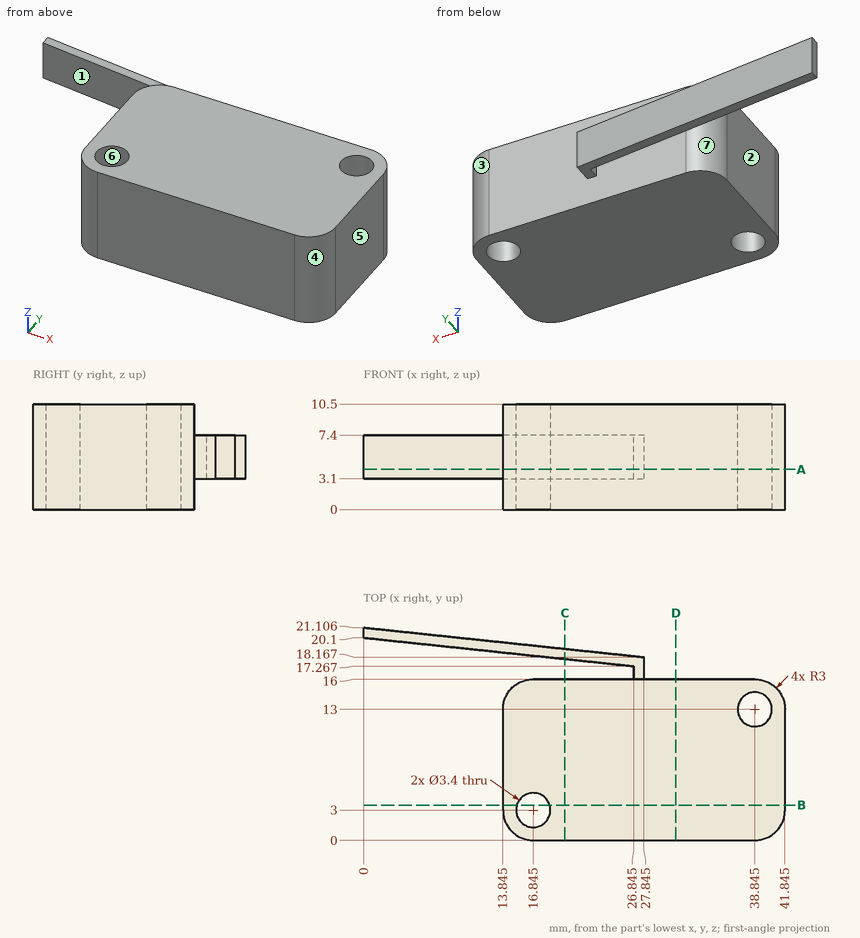
The figure shows three views and two pictorial views of one solid part (mm, origin at its lowest corner). Answer the questions. A direction names the side the tool comes from. Give positions to 0.01 mm unless a question says otherwise; leave off trailing zeros. Write each loop counter-clockwise with the first axis right and the second up, starting at its lowest first coordinate (ties: lowest second). Pieces come first, ordered by that corner, then holes. Notation, with made-up numbers: (-32, -24.75) -> (6, -24.75) arc R28 ccw to (6, -2.75) -> close; hole circle Ø9 at (-8, 48.25). An arc over 180 degrees is marked (long way). Answer as a JSON object with one key per item and string values.
1) Straight lines are drawn through the part: probe 1 along Y at (x, z) = (37, 4.5); probe 2 along Y at (x, z) = (26.5, 7); probe 3 along X at (y, z) = (13.75, 7.75). For each, find the intervals that lie inside material, in ascending order. Write a range as from..to.
Findings below:
{"probe 1": "y = 0..16", "probe 2": "y = 0..16, 17.3..18.31", "probe 3": "x = 13.94..37.32, 40.37..41.75"}
2) Section A-A on z = 4 is taken. Write down the section's boundary in (x, y) (1 decimal).
Findings below:
{"outline": "(0, 20.1) -> (26.8, 17.3) -> (26.8, 16) -> (16.8, 16) arc R3 ccw to (13.8, 13) -> (13.8, 3) arc R3 ccw to (16.8, 0) -> (38.8, 0) arc R3 ccw to (41.8, 3) -> (41.8, 13) arc R3 ccw to (38.8, 16) -> (27.8, 16) -> (27.8, 18.2) -> (0, 21.1) -> close; hole circle Ø3.4 at (16.8, 3); hole circle Ø3.4 at (38.8, 13)"}
3) Section D-D on x = 31 is taken. Write down the section's boundary in (y, z).
Findings below:
{"outline": "(0, 0) -> (16, 0) -> (16, 10.5) -> (0, 10.5) -> close"}
4) Section C-C on x = 20 is taken. Write down the section's boundary in (y, z) (1 decimal), then the cut area to 3 significant figures.
Findings below:
{"outline": "(0, 0) -> (16, 0) -> (16, 10.5) -> (0, 10.5) -> close; (18, 3.1) -> (19, 3.1) -> (19, 7.4) -> (18, 7.4) -> close", "area": "172 mm^2"}
5) Section B-B on y = 3.5 is taken. Write down the section's boundary in (x, z) (1 decimal).
Findings below:
{"outline": "(13.8, 0) -> (15.2, 0) -> (15.2, 10.5) -> (13.8, 10.5) -> close; (18.5, 0) -> (41.8, 0) -> (41.8, 10.5) -> (18.5, 10.5) -> close"}
6) A tool of negligible diameter and unlimited length cuts with its end or side. For the marked faces 1, 2 and 3, from which of +Z, -Z, +X, -X, +Y, -Y can it reach the whole face along a straight path? Write none if from no direction.
Findings below:
{"face 1": "+Z, -Z, -X", "face 2": "+Z, -Z, -X, -Y", "face 3": "+Z, -Z, +X, +Y"}
7) For a pull along Y with two mould halves and no side action, classify the marked faces 4, 5, 6 and 7 as pulls with the +Y half, pulls with the -Y half, needs draft (parallel to the pull), parting line crosses it, or undercut.
Findings below:
{"face 4": "pulls with the -Y half", "face 5": "needs draft", "face 6": "undercut", "face 7": "undercut"}
8) Flat-ended cylindrical pins translate along their axes: pin 1 Ø4 at (x, y) = (14, 19.5) entering from +Z; pin 2 Ø1.5 at (x, y) = (19.5, 17.5) entering from -Z; pin 3 Ø2.5 at (y, z) = (17, 5) entering from +X (1 decimal); pin 4 Ø3 at (x, y) = (38.85, 13) entering from +Z. Find the tip coordinate at first contact, or state that the pin passes through.
Findings below:
{"pin 1": "stops at z = 7.4", "pin 2": "stops at z = 3.1", "pin 3": "stops at x = 40", "pin 4": "passes through"}
